```python
from build123d import *

# Parameters (mm, degrees)
SKETCH1_W           = 9.525
SKETCH1_H           = 12.7
BOSS_EXTRUDE1_DEPTH = 92.075
SKETCH2_W           = 3.175
SKETCH2_H           = 12.7
CUT_EXTRUDE1_DEPTH  = 168.784366554
SKETCH4_R           = 3.175
CUT_EXTRUDE3_DEPTH  = 99.934266019


with BuildPart() as part:
    # Sketch1 → Boss-Extrude1 (new body)
    with BuildSketch(Plane.XY):
        with Locations((134.924643413, -28.57073514)):
            Rectangle(SKETCH1_W, SKETCH1_H)
    extrude(amount=BOSS_EXTRUDE1_DEPTH)

    # Sketch2 → Cut-Extrude1 (cut, through all)
    with BuildSketch(Plane(origin=(0, -22.22073514, 0), x_dir=(1, 0, 0), z_dir=(0, 1, 0))):
        with Locations((134.924643413, -85.725)):
            Rectangle(SKETCH2_W, SKETCH2_H)
        with Locations((134.924643413, -6.35)):
            Rectangle(SKETCH2_W, SKETCH2_H)
    extrude(amount=-CUT_EXTRUDE1_DEPTH, mode=Mode.SUBTRACT)

    # Sketch4 → Cut-Extrude3 (cut, through all)
    with BuildSketch(Plane(origin=(139.687143413, 0, 0), x_dir=(0, 0, -1), z_dir=(1, 0, 0))):
        with Locations((-6.35, -28.57073514)):
            Circle(SKETCH4_R)
        with BuildLine():
            Line((0, -22.22073514), (-6.35, -22.22073514))
            ThreePointArc((-6.35, -22.22073514), (-1.859871939, -24.080607079), (0, -28.57073514))
            Line((0, -28.57073514), (0, -22.22073514))
        make_face()
        with BuildLine():
            Line((0, -34.92073514), (0, -28.57073514))
            ThreePointArc((0, -28.57073514), (-1.859871939, -33.060863201), (-6.35, -34.92073514))
            Line((-6.35, -34.92073514), (0, -34.92073514))
        make_face()
        with Locations((-85.725, -28.57073514)):
            Circle(SKETCH4_R)
        with BuildLine():
            ThreePointArc((-92.075, -28.57073514), (-90.215128061, -24.080607079), (-85.725, -22.22073514))
            Line((-85.725, -22.22073514), (-92.075, -22.22073514))
            Line((-92.075, -22.22073514), (-92.075, -28.57073514))
        make_face()
        with BuildLine():
            ThreePointArc((-85.725, -34.92073514), (-90.215128061, -33.060863201), (-92.075, -28.57073514))
            Line((-92.075, -28.57073514), (-92.075, -34.92073514))
            Line((-92.075, -34.92073514), (-85.725, -34.92073514))
        make_face()
    extrude(amount=-CUT_EXTRUDE3_DEPTH, mode=Mode.SUBTRACT)


solid = part.part
```
For this review, take the finished solid that the model builds, in its own axes (mm). A direction names the side the tool comes from. Give positions to 0.01 mm unless a question says otherwise; leave off trailing zeros. Loops run counter-clockwise (first coordinate to the right, second up) from the corner with the lowest first, then second, coordinate; pieces in that order, holes last. Notation, with made-up numbers: M -16.75,-13 L 42.25,-13 A26 ccw 42.25,26 Z; hole C 3,41.25 d2. An arc over 180 degrees is marked long. One line per item, written item: value. Start each with the question number.
Q1. Add section C-C (y = -24). Give the boundary of the cut face in (x, z) (3 decimals).
Q2. Add section D-D (x = 134.25). Give the boundary of the cut face in (y, z) (3 decimals), and give its area (3 significant figures).
Q3. For L1, parallel to X at y = -27.75, z = 9.5; L2, parallel to Y at x = 132.6, z = 6.35; L3, parallel to Z at x = 136, y = -33.5 (3 decimals), list the stretches that pass through material, from the lowest coordinate up.
Q4. Add section A-A (x = 138.25). Give the boundary of the cut face in (y, z) (3 decimals), and give its area (3 significant figures).
Q5. Draft analysis for pull direction X (two halves, no side actions). For faces 4 (the face through (130.162, -29, 45)), 5 (the face through (139.687, -29, 45)), 6 (the face through (133.337, -28, 82)), state which applies: released by +X, released by -X, zero draft, split by the parting line, or undercut.
Q6. Machinability: for faces 1 (the face through (131.772, -30.503, 88.245)), 2 (the face through (136.512, -26, 9)), 3 (the face through (136.512, -28, 82)), which of the approach directions +Z, -Z, +X, -X, +Y, -Y give a long, thin tool a straight path to every point of the face, cutting with its end or side? Answer none if there is none.
Q7. Add section B-B (z = 87). Give the boundary of the cut face in (x, y).
Q8. Clearance check with flat-ended pins moving along their axes: pin 1 Ø1 at (x, y) = (134.5, -31.5) entering from -Z; pin 2 Ø2.5 at (x, y) = (134.5, -29.5) entering from +Z. State where each tip first meets the part, or that it passes through.
Reply:
1. outline: M 130.162,1.942 L 133.337,1.942 L 133.337,12.7 L 136.512,12.7 L 136.512,1.942 L 139.687,1.942 L 139.687,90.133 L 136.512,90.133 L 136.512,79.375 L 133.337,79.375 L 133.337,90.133 L 130.162,90.133 Z
2. outline: M -34.921,12.7 L -22.221,12.7 L -22.221,79.375 L -34.921,79.375 Z
2. area: 847 mm²
3. L1: 130.16 to 133.34, 136.51 to 139.69
3. L2: -34.92 to -31.75, -25.4 to -22.22
3. L3: 12.7 to 79.375
4. outline: M -34.921,6.35 A6.35 ccw -22.221,6.35 L -22.221,85.725 A6.35 ccw -34.921,85.725 Z; hole C -28.571,6.35 d6.35; hole C -28.571,85.725 d6.35
4. area: 1,070 mm²
5. face 4: released by -X
5. face 5: released by +X
5. face 6: undercut
6. face 1: +X, -X
6. face 2: -Z, +Y, -Y
6. face 3: +Z, +Y, -Y
7. outline: M 130.16,-34.79 L 133.34,-34.79 L 133.34,-31.48 L 130.16,-31.48 Z; M 130.16,-25.66 L 133.34,-25.66 L 133.34,-22.35 L 130.16,-22.35 Z; M 136.51,-34.79 L 139.69,-34.79 L 139.69,-31.48 L 136.51,-31.48 Z; M 136.51,-25.66 L 139.69,-25.66 L 139.69,-22.35 L 136.51,-22.35 Z
8. pin 1: z = 12.7
8. pin 2: z = 92.06
